The model under review builds one solid part; all positions refer to its coordinate system, in mm. A direction names the side the tool comes from. Round coordinates to 2 decimals unless told otherwise and drop trailing zeros. Loops run counter-clockwise (first coordinate to the right, second up) from the corner with the lowest first, then second, coordinate; pieces in that order, holes last. Notation, with made-up numbers: M 37.5,-9 L 68.5,-9 A15 ccw 68.5,18 Z; hole C -25,15 d9. An arc over 180 degrees is marked long. Return JSON: item names as keys, results as strings. Group by question number.
Q1. Draft analysis for pull direction X (two halves, no side actions). For faces 1 (the face through (1, 44, 9.525)), 2 (the face through (60.325, 0, 50)), 3 (the face through (94.996, -19, 62)), 4 (the face through (46.919, -0.356, 48.964)), state which applies: pulls with the +X half, pulls with the -X half, needs draft (parallel to the pull), parting line crosses it, or undercut.
Q2. Consider section A-A (x = 81.5). State the section outline as (y, z) points (3 decimals), and give its area (3 significant figures).
Q3. To check wall thickness, follow line 1 along Z through (x, y) = (99, -8) (3 decimals); line 2 along X through (y, z) = (-33, -1) (3 decimals); line 3 along Y through (x, z) = (29.5, 43.5). State the ranges of each line that lie inside material, in increasing order.
Q4. Consider section B-B (y = 31). State the section outline as (x, z) points (3 decimals).
Q5. Clearance check with flat-ended pins moving along their axes: pin 1 Ø6.5 at (y, z) = (-16, 60.5) entering from +X; pin 2 Ø3.5 at (y, z) = (-19.5, 74) entering from +X (3 decimals); pin 3 Ø10 at (y, z) = (1.5, 0.5) entering from -X (3 decimals). State where each tip first meets the part, or that it passes through.
Q6. For faces 5 (the face through (85, 0, 47.625)), 6 (the face through (12, 25.4, 44)), 7 (the face through (1, -45, 9.525)), 8 (the face through (60.325, -19, 74)), list the 3-axis set-ups (+Z, -Z, +X, -X, +Y, -Y) from which the entire face can be reached by the end or side of a thin tool; tool diameter is ignored.
from build123d import *

# Parameters (mm, degrees)
F1_DEPTH = 63.5
F2_DEPTH = 25.4
F3_DEPTH = 25.4
F4_DEPTH = 25.4
F5_DEPTH = 12.7


with BuildPart() as f1:
    # F0 (on Front) → F1 (new body, symmetric)
    with BuildSketch(Plane.XZ):
        Polygon((22.225, 9.525), (-41.275, 9.525), (-41.275, -9.525), (41.275, -9.525), (41.275, 9.525), align=None)
    extrude(amount=F1_DEPTH, both=True)

    # F0 (on Front) → F2 (join, symmetric)
    with BuildSketch(Plane.XZ):
        with BuildLine():
            Line((22.225, 36.82567), (22.225, 9.525))
            Line((22.225, 9.525), (41.275, 9.525))
            Line((41.275, 9.525), (41.275, 36.82567))
            ThreePointArc((41.275, 36.82567), (47.069933, 49.089759), (60.224024, 52.4002))
            Line((60.224024, 52.4002), (60.325, 52.4002))
            Line((60.325, 52.4002), (60.325, 71.606052))
            ThreePointArc((60.325, 71.606052), (33.60357, 62.619491), (22.225, 36.82567))
        make_face()
    extrude(amount=F2_DEPTH, both=True)

    # F0 (on Front) → F3 (join, symmetric)
    with BuildSketch(Plane.XZ):
        with BuildLine():
            ThreePointArc((61.72138, 71.4502), (61.023974, 71.535149), (60.325, 71.606052))
            Line((60.325, 71.606052), (60.325, 52.4002))
            Line((60.325, 52.4002), (94.995893, 52.4002))
            Line((94.995893, 52.4002), (94.995893, 71.4502))
            Line((94.995893, 71.4502), (61.72138, 71.4502))
        make_face()
    extrude(amount=F3_DEPTH, both=True)

    # F0 (on Front) → F4 (join, symmetric)
    with BuildSketch(Plane.XZ):
        with BuildLine():
            add(Edge.make_bspline(
                [(-41.275, 9.525), (-42.333655, 75.119734), (0, 76.560877), (60.325, 76.2)],
                knots=[0, 0, 0, 0, 121.524136, 121.524136, 121.524136, 121.524136], degree=3))
            Line((-41.275, 9.525), (22.225, 9.525))
            Line((22.225, 9.525), (22.225, 36.82567))
            ThreePointArc((22.225, 36.82567), (33.60357, 62.619491), (60.325, 71.606052))
            Line((60.325, 71.606052), (60.325, 76.2))
        make_face()
    extrude(amount=F4_DEPTH, both=True)

    # F0 (on Front) → F5 (join, symmetric)
    with BuildSketch(Plane.XZ):
        with BuildLine():
            Line((111.125, 76.2), (60.325, 76.2))
            Line((60.325, 76.2), (60.325, 71.606052))
            ThreePointArc((60.325, 71.606052), (61.023974, 71.535149), (61.72138, 71.4502))
            Line((61.72138, 71.4502), (94.995893, 71.4502))
            Line((94.995893, 71.4502), (94.995893, 52.4002))
            Line((94.995893, 52.4002), (60.325, 52.4002))
            Line((60.325, 52.4002), (60.325, 47.625))
            Line((60.325, 47.625), (111.125, 47.625))
            Line((111.125, 47.625), (111.125, 76.2))
        make_face()
    extrude(amount=F5_DEPTH, both=True)


solid = f1.part
Values:
{
 "1": {"face 1": "needs draft", "face 2": "undercut", "face 3": "pulls with the +X half", "face 4": "undercut"},
 "2": {"outline": "M -25.4,52.4 L -12.7,52.4 L -12.7,47.625 L 12.7,47.625 L 12.7,52.4 L 25.4,52.4 L 25.4,71.45 L 12.7,71.45 L 12.7,76.2 L -12.7,76.2 L -12.7,71.45 L -25.4,71.45 Z", "area": "1,210 mm2"},
 "3": {"line 1": "z = 47.625 to 76.2", "line 2": "x = -41.275 to 41.275", "line 3": "y = -25.4 to 25.4"},
 "4": {"outline": "M -41.275,-9.525 L 41.275,-9.525 L 41.275,9.525 L -41.275,9.525 Z"},
 "5": {"pin 1": "stops at x = 95", "pin 2": "stops at x = 60.325", "pin 3": "stops at x = -41.275"},
 "6": {"face 5": "-Z, +X, +Y, -Y", "face 6": "+Z, +X, -X, +Y", "face 7": "+Z, +X, -X, -Y", "face 8": "+Z, +X, -Y"}
}
